Can you work these out from the model? Positions are in its coordinate system, mm. A direction names the side the tool comes from. Coordinates: 2 decimals unless noted, no trailing zeros. Loops run counter-clockwise (first coordinate to the right, second up) from the corner with the lowest first, then second, coordinate; pieces in that order, holes last. Notation, with made-up numbers: M -6.75,65.25 L 13.25,65.25 A19 cw 13.25,102.25 Z; hole C -38.75,-7.5 d8. An arc over 180 degrees is marked long. Answer as a JSON object with one key per item and string values. Group by question number.
Item 1: Suppose I cut it at D-D (x = -169.5). Write out the boundary of the cut face in (y, z).
Item 2: Suppose I cut it at A-A (x = -26). Write out the boundary of the cut face in (y, z), then the cut area to 3 significant figures.
Item 3: We'd pull the mould along X, two halves only. Please class faces 1 (the flat face through (-44, -508, -19)), 2 (the flat face through (86.449, -250.444, -35.224)), 3 (the flat face through (-44, -25.4, -13)): +X half, -X half, draft (parallel to the pull), parting line (faces both ways), or undercut.
Item 4: If I drill on line 1 (X direction, y = -93, z = -1); line 2 (Y direction, x = -116, z = 5.5); line 3 (Z direction, x = -143, y = -399), over which ranges is the centre line in solid material (lowest first)?
Item 5: I'm going to push flat-ended pins straight in: pin 1 Ø6 at (y, z) = (-314.5, -30.5) entering from -X; pin 2 Ø3 at (y, z) = (-208.5, -20.5) entering from +X; pin 3 Ø6 at (x, y) = (37.5, -162) entering from +Z; pin 4 Ø12 at (y, z) = (-150.5, -13.5) entering from +X. Where does each tip first touch, or does it pass through?
Item 6: Suppose I cut it at B-B (z = -36.5). Write out the boundary of the cut face in (x, y).
Item 7: Suppose I cut it at C-C (y = -123). Write out the boundary of the cut face in (x, z), then the cut area to 3 significant figures.
Item 8: Which directions (+Z, -Z, +X, -X, +Y, -Y) give clear straight access to the entire face, cutting with the end or side of a thin tool? Please do faces 4 (the flat face through (-161.483, -250.8, -26.13)), 5 (the flat face through (-44, 0, -19)).
```python
from build123d import *

# Parameters (mm, degrees)
F0_W     = 12.7
F0_H     = 25.4
F0_W_2   = 203.2
F0_H_2   = 12.7
F1_DEPTH = 508
F3_DEPTH = 25.4
F5_DEPTH = 25.4


with BuildPart() as f1:
    # F0 (on Front) → F1 (new body)
    with BuildSketch(Plane.XZ):
        with Locations((102.376167, 4.548111)):
            Rectangle(F0_W, F0_H)
        Polygon((104.891275, -17.245835), (96.026167, -8.151889), (59.65038, -43.612319), (68.515488, -52.706266), align=None)
        Polygon((108.726167, -8.151889), (96.026167, -8.151889), (104.891275, -17.245835), align=None)
        with Locations((-41.94962, -49.962319)):
            Rectangle(F0_W_2, F0_H_2)
        Polygon((68.515488, -52.706266), (59.65038, -43.612319), (59.65038, -56.312319), align=None)
        Polygon((-152.414727, -52.706266), (-143.54962, -43.612319), (-179.925407, -8.151889), (-188.790514, -17.245835), align=None)
        Polygon((-143.54962, -56.312319), (-143.54962, -43.612319), (-152.414727, -52.706266), align=None)
        with Locations((-186.275407, 4.548111)):
            Rectangle(F0_W, F0_H)
        Polygon((-188.790514, -17.245835), (-179.925407, -8.151889), (-192.625407, -8.151889), align=None)
    extrude(amount=F1_DEPTH)

    # F2 (on Front) → F3 (join)
    with BuildSketch(Plane.XZ):
        Polygon((96.026167, 17.248111), (-179.925407, 17.248111), (-179.925407, -8.151889), (-143.54962, -43.612319), (59.65038, -43.612319), (96.026167, -8.151889), align=None)
    extrude(amount=F3_DEPTH)

    # F4 (on face) → F5 (join)
    with BuildSketch(Plane.XZ.offset(508)):
        Polygon((96.026167, 17.248111), (-179.925407, 17.248111), (-179.925407, -8.151889), (-143.54962, -43.612319), (59.65038, -43.612319), (96.026167, -8.151889), align=None)
    extrude(amount=-F5_DEPTH)


solid = f1.part
```
From the geometry:
{
 "1": {"outline": "M -508,-36.05 L 0,-36.05 L 0,17.25 L -25.4,17.25 L -25.4,-18.31 L -482.6,-18.31 L -482.6,17.25 L -508,17.25 Z"},
 "2": {"outline": "M -508,-56.31 L 0,-56.31 L 0,17.25 L -25.4,17.25 L -25.4,-43.61 L -482.6,-43.61 L -482.6,17.25 L -508,17.25 Z", "area": "9,540 mm2"},
 "3": {"face 1": "draft", "face 2": "+X half", "face 3": "undercut"},
 "4": {"line 1": "-192.63 to -179.93, 96.03 to 108.73", "line 2": "-508 to -482.6, -25.4 to 0", "line 3": "-56.31 to -43.61"},
 "5": {"pin 1": "x = -178.27", "pin 2": "x = 103.09", "pin 3": "z = -43.61", "pin 4": "x = 108.73"},
 "6": {"outline": "M -169.04,-508 L 85.14,-508 L 85.14,0 L -169.04,0 Z; hole M -150.85,-482.6 L 66.95,-482.6 L 66.95,-25.4 L -150.85,-25.4 Z"},
 "7": {"outline": "M -192.63,-8.15 L -188.79,-17.25 L -152.41,-52.71 L -143.55,-56.31 L 59.65,-56.31 L 68.52,-52.71 L 104.89,-17.25 L 108.73,-8.15 L 108.73,17.25 L 96.03,17.25 L 96.03,-8.15 L 59.65,-43.61 L -143.55,-43.61 L -179.93,-8.15 L -179.93,17.25 L -192.63,17.25 Z", "area": "4,740 mm2"},
 "8": {"face 4": "+Z", "face 5": "+Z, -Z, +X, -X, +Y"}
}
